Work out the finished part from the listing and answer in its coordinate system (mm). A direction names the side the tool comes from. Give positions to 0.01 mm unless a question says otherwise; leave off trailing zeros. Order: outer loops, then holes, each group sorted by start corner. A loop starts at its lowest first (then second) coordinate and runs counter-clockwise, first axis right, second up. Notation, with made-up numbers: (-3.5, 70) -> (13.5, 70) arc R14 ccw to (13.5, 97) -> close; hole circle Ø10 at (49.5, -14). An arc over 180 degrees is marked (long way). Use a Markdown table: item, result. Add a question column.
```python
from build123d import *

# Parameters (mm, degrees)
F0_W     = 25.2222
F0_H     = 23.876
F0_R     = 1.27
F1_DEPTH = 1.016
F2_W     = 8.001
F2_H     = 8.001
F3_DEPTH = 5.08
F4_W     = 20.32
F4_H     = 5.461
F5_DEPTH = 2.54


with BuildPart() as f1:
    # F0 (on Front) → F1 (new body)
    with BuildSketch(Plane.XZ):
        Rectangle(F0_W, F0_H)
        with Locations((-10.3251, -9.779)):
            Circle(F0_R, mode=Mode.SUBTRACT)
        with Locations((10.3251, -9.779)):
            Circle(F0_R, mode=Mode.SUBTRACT)
        with Locations((-10.3251, 2.54)):
            Circle(F0_R, mode=Mode.SUBTRACT)
        with Locations((10.3251, 2.54)):
            Circle(F0_R, mode=Mode.SUBTRACT)
    extrude(amount=-F1_DEPTH)

    # F2 (on face) → F3 (join)
    with BuildSketch(Plane.XZ):
        with Locations((0, 2.4765)):
            Rectangle(F2_W, F2_H)
    extrude(amount=F3_DEPTH)

    # F4 (on face) → F5 (join)
    with BuildSketch(Plane(origin=(0, 1.016, 0), x_dir=(-1, 0, 0), z_dir=(0, 1, 0))):
        with Locations((0, 9.2075)):
            Rectangle(F4_W, F4_H)
    extrude(amount=F5_DEPTH)


solid = f1.part
```
1) The part is cut by section A-A, the plane z = 2.54. Determine the outline of the cut face in (x, y), then the cut area to 3 significant figures.
2) Determine the mould class of faces 5 (the cylindrical face through (11.498, 0.501, 2.054)), 6 (the flat face through (-0.2, 0.5, -11.938)), 7 (the flat face through (10.16, 2, 9)) for opening direction Z: released by +Z, released by -Z, zero draft, split by the parting line, or undercut.
3) Straight lines are drawn through the part: line 1 (Z direction, x = -0.75, y = 3); line 2 (Y direction, x = -7.5, z = -4); line 3 (X direction, y = 2, z = 8). For each, find the intervals that lie inside material, in ascending order.
4) Flat-ended cylindrical pins translate along their axes: pin 1 (1.5 mm diameter, centred on x = -10.33, z = 2.54, fed in from -Y); pin 2 (1.3 mm diameter, centred on y = 2, z = 8, fed in from +X); pin 3 (4 mm diameter, centred on y = -3, z = 1.5, fed in from +X); pin 4 (0.8 mm diameter, centred on y = 2, z = 10, fed in from -X). Find the tip coordinate at first contact, or state that the pin passes through.
5) The part is cut by section C-C, the plane y = -4. Determine the outline of the cut face in (x, z), then the cut area to 3 significant figures.
6) The part is cut by section D-D, the plane z = -4.5. Determine the outline of the cut face in (x, y), then the cut area to 3 significant figures.
7) Which of the six approach directions +Z, -Z, +X, -X, +Y, -Y give full straight-line access (tool end or side, diameter ignored) to faces 1 (the flat face through (0, 2, 6.477)), 2 (the flat face through (-4, -3, 2)), 3 (the flat face through (-10.16, 2, 9)), 4 (the flat face through (0, -3, -1.524))?
8) The part is cut by section B-B, the plane x = 2.75. Determine the outline of the cut face in (y, z), then the cut area to 3 significant figures.
A:
| question | item | result |
|---|---|---|
| 1 | outline | (-12.61, 0) -> (-11.6, 0) -> (-11.6, 1.02) -> (-12.61, 1.02) -> close; (-9.06, 0) -> (-4, 0) -> (-4, -5.08) -> (4, -5.08) -> (4, 0) -> (9.06, 0) -> (9.06, 1.02) -> (-9.06, 1.02) -> close; (11.6, 0) -> (12.61, 0) -> (12.61, 1.02) -> (11.6, 1.02) -> close |
| 1 | area | 61.1 mm^2 |
| 2 | face 5 | undercut |
| 2 | face 6 | released by -Z |
| 2 | face 7 | zero draft |
| 3 | line 1 | 6.48 to 11.94 |
| 3 | line 2 | 0 to 1.02 |
| 3 | line 3 | -10.16 to 10.16 |
| 4 | pin 1 | through |
| 4 | pin 2 | x = 10.16 |
| 4 | pin 3 | x = 4 |
| 4 | pin 4 | x = -10.16 |
| 5 | outline | (-4, -1.52) -> (4, -1.52) -> (4, 6.48) -> (-4, 6.48) -> close |
| 5 | area | 64.0 mm^2 |
| 6 | outline | (-12.61, 0) -> (12.61, 0) -> (12.61, 1.02) -> (-12.61, 1.02) -> close |
| 6 | area | 25.6 mm^2 |
| 7 | face 1 | -Z, +X, -X, +Y |
| 7 | face 2 | +Z, -Z, -X, -Y |
| 7 | face 3 | +Z, -Z, -X, +Y |
| 7 | face 4 | -Z, +X, -X, -Y |
| 8 | outline | (-5.08, -1.52) -> (0, -1.52) -> (0, -11.94) -> (1.02, -11.94) -> (1.02, 6.48) -> (3.56, 6.48) -> (3.56, 11.94) -> (0, 11.94) -> (0, 6.48) -> (-5.08, 6.48) -> close |
| 8 | area | 78.8 mm^2 |
